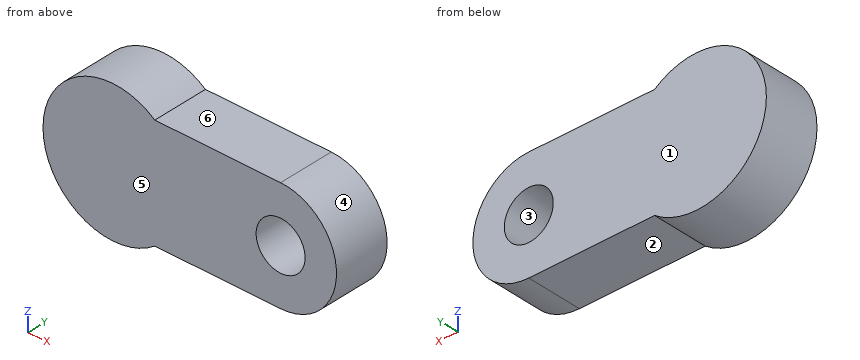
from build123d import *

# Parameters (mm, degrees)
F0_R     = 11.1125
F1_DEPTH = 25.4


with BuildPart() as f1:
    # F0 (on Front) → F1 (new body)
    with BuildSketch(Plane.XZ):
        with BuildLine():
            ThreePointArc((-25.493373, -25.4), (-16.145309, -14.199032), (-12.793373, 0))
            ThreePointArc((-12.793373, 0), (-16.145309, 14.199032), (-25.493373, 25.4))
            ThreePointArc((-25.493373, 25.4), (-76.293373, 0), (-25.493373, -25.4))
        make_face()
        with BuildLine():
            ThreePointArc((-25.493373, 25.4), (-16.145309, 14.199032), (-12.793373, 0))
            ThreePointArc((-12.793373, 0), (-16.145309, -14.199032), (-25.493373, -25.4))
            Line((-25.493373, -25.4), (31.656627, -25.4))
            ThreePointArc((31.656627, -25.4), (57.056627, 0), (31.656627, 25.4))
            Line((31.656627, 25.4), (-25.493373, 25.4))
        make_face()
        with Locations((31.656627, 0)):
            Circle(F0_R, mode=Mode.SUBTRACT)
    extrude(amount=F1_DEPTH)


solid = f1.part
Geometry: final body of the model. Coordinates: model frame, mm. Face numbers are marked on the shaded views. A direction names the side the tool comes from. Give positions to 0.01 mm unless a question says otherwise; leave off trailing zeros. Loops run counter-clockwise (first coordinate to the right, second up) from the corner with the lowest first, then second, coordinate; pieces in that order, holes last. Notation, with made-up numbers: (70.25, -9.75) - (121.25, -9.75) arc R19 ccw to (121.25, -2.75) - close; hole circle Ø11 at (8.25, 42). An arc over 180 degrees is marked (long way). One line per question, with ' | ' between items. Start each with the question number.
(1) Section query C-C on z = -7.5. Return loops of the section in (x, y).
(2) Section query A-A on z = 0. Return loops of the section in (x, y), then the cut area to 3 significant figures.
(3) Pull-direction query (Z, two-part tool) for the marked faces 3, 4, 5 and 6; classes: released by +Z, released by -Z, zero draft, split by the parting line, or undercut.
(4) Ray query, line 1 (Z direction, x = 13.5, y = -13.5); line 2 (X direction, y = -1.25, z = -5); line 3 (X direction, y = -10.5, z = 9). Return the intervals inside material, ascending. Write a range as from..to.
(5) Reachability of the marked faces 1 and 2 from +Z, -Z, +X, -X, +Y, -Y: full face, straight path, thin tool, end or side. Return the list, or none.
(6) Contact query for flat-ended pins moving along their axis: pin 1 (10 mm diameter, centred on y = -20.5, z = 12, fed in from -X); pin 2 (1 mm diameter, centred on x = 40.5, z = 24, fed in from -Y); pin 3 (3 mm diameter, centred on x = -2, y = -10.5, fed in from -Z); pin 4 (7.5 mm diameter, centred on x = -3, y = -10.5, fed in from +Z). Output: stop coordinate, or through.
(7) Section query D-D on x = -14. Return loops of the section in (y, z), then the cut area to 3 significant figures.
The answers:
1) outline: (-75.39, -25.4) - (23.46, -25.4) - (23.46, 0) - (-75.39, 0) - close; (39.86, -25.4) - (55.92, -25.4) - (55.92, 0) - (39.86, 0) - close
2) outline: (-76.29, -25.4) - (20.54, -25.4) - (20.54, 0) - (-76.29, 0) - close; (42.77, -25.4) - (57.06, -25.4) - (57.06, 0) - (42.77, 0) - close | area: 2,820 mm2
3) face 3: undercut | face 4: split by the parting line | face 5: zero draft | face 6: released by +Z
4) line 1: -25.4..25.4 | line 2: -75.9..21.73, 41.58..56.56 | line 3: -74.99..25.14, 38.17..55.41
5) face 1: +Z, -Z, +X, -X, +Y | face 2: -Z, +X, +Y, -Y
6) pin 1: x = -75.51 | pin 2: y = -25.4 | pin 3: z = -25.4 | pin 4: z = 25.4
7) outline: (-25.4, -25.4) - (0, -25.4) - (0, 25.4) - (-25.4, 25.4) - close | area: 1,290 mm2
